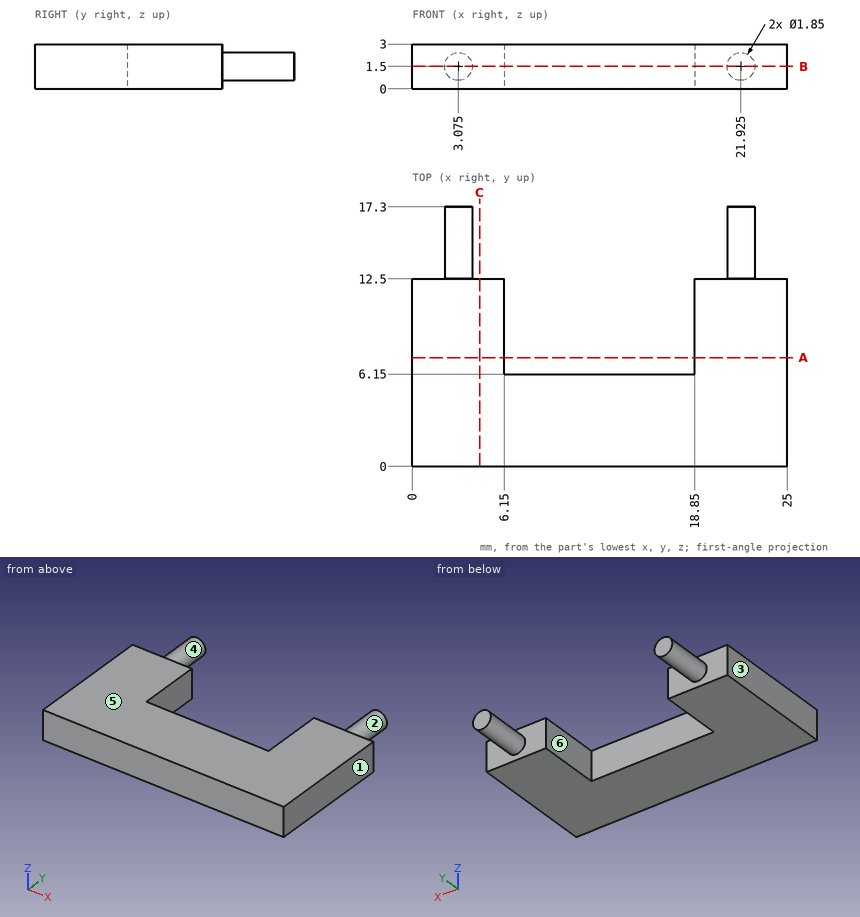
Print and shaded views of the part. All mm, measured from the part's lowest x, y and z. A direction names the side the tool comes from. Give positions to 0.01 mm unless a question says otherwise; leave off trailing zeros. Loops run counter-clockwise (first coordinate to the right, second up) from the corner with the lowest first, then second, coordinate; pieces in that order, holes last. Notation, with made-up numbers: (18.25, -4) - (22.25, -4) arc R28 ccw to (22.25, 16) - close; hole circle Ø3 at (-39.5, 19). An arc over 180 degrees is marked (long way). Use a Markdown table: item, result.
(1) Band-saw the part on A-A (y = 7.25). Give the cut face in (x, z), and give its area (3 significant figures).
Taken from the geometry:
| item | result |
|---|---|
| outline | (0, 0) - (6.15, 0) - (6.15, 3) - (0, 3) - close; (18.85, 0) - (25, 0) - (25, 3) - (18.85, 3) - close |
| area | 36.9 mm2 |
(2) Drop a flat-ended pin along its axis: pin 1 Ø0.9 at (x, z) = (11, 1.5) entering from +Y. Give the stop position or say it passes through.
Taken from the geometry:
| item | result |
|---|---|
| pin 1 | y = 6.15 |
(3) Wall check: line 1 along X through (y, z) = (6.5, 0.7); line 2 along X through (y, z) = (14.75, 1.45); line 3 along Y through (x, z) = (5.25, 1.8). Give the ranges that are in metal, low to high.
Taken from the geometry:
| item | result |
|---|---|
| line 1 | 0 to 6.15, 18.85 to 25 |
| line 2 | 2.15 to 4, 21 to 22.85 |
| line 3 | 0 to 12.5 |
(4) Band-saw the part on B-B (z = 1.5). Give the cut face in (x, y).
Taken from the geometry:
| item | result |
|---|---|
| outline | (0, 0) - (25, 0) - (25, 12.5) - (22.85, 12.5) - (22.85, 17.3) - (21, 17.3) - (21, 12.5) - (18.85, 12.5) - (18.85, 6.15) - (6.15, 6.15) - (6.15, 12.5) - (4, 12.5) - (4, 17.3) - (2.15, 17.3) - (2.15, 12.5) - (0, 12.5) - close |
(5) Band-saw the part on C-C (x = 4.5). Give the cut face in (y, z).
Taken from the geometry:
| item | result |
|---|---|
| outline | (0, 0) - (12.5, 0) - (12.5, 3) - (0, 3) - close |
(6) Pull direction X, two halves, no side cores. Call the marked faces 1, 2 and 3: +X half, -X half, draft (parallel to the pull), parting line (faces both ways), or undercut.
Taken from the geometry:
| item | result |
|---|---|
| face 1 | +X half |
| face 2 | undercut |
| face 3 | -X half |
(7) Which spindle directions (+Z, -Z, +X, -X, +Y, -Y) get a long thin tool onto all of the face, cutting with end or side? Do the marked faces 4, 5 and 6. Say none if no direction does.
Taken from the geometry:
| item | result |
|---|---|
| face 4 | +Y |
| face 5 | +Z, +X, -X, +Y, -Y |
| face 6 | +Z, -Z, +Y |
